from build123d import *

# Parameters (mm, degrees)
F1_DEPTH = 100
F2_DEPTH = 25
F3_DEPTH = 50
F5_DEPTH = 12.5
F6_R     = 15


with BuildPart() as f1:
    # F0 (on Front) → F1 (new body, symmetric)
    with BuildSketch(Plane.XZ):
        Polygon((-50, 25), (-50, -25), (50, -25), (50, 25), (19.234454, 25), (-0.765546, 25), align=None)
    extrude(amount=F1_DEPTH, both=True)

    # F0 (on Front) → F2 (join, symmetric)
    with BuildSketch(Plane.XZ):
        with BuildLine():
            Line((-0.765546, 60), (-0.765546, 25))
            Line((-0.765546, 25), (19.234454, 25))
            Line((19.234454, 25), (19.234454, 60))
            ThreePointArc((19.234454, 60), (37.397461, 98.553935), (78.690689, 109.097654))
            Line((78.690689, 109.097654), (118.690689, 109.097654))
            Line((118.690689, 109.097654), (118.690689, 129.097654))
            Line((118.690689, 129.097654), (80.437767, 129.097654))
            add(Edge.make_bspline(
                [(53.363976, 128.17718), (62.022985, 128.828118), (71.068506, 129.097654), (80.437767, 129.097654)],
                knots=[145.637672, 145.637672, 145.637672, 145.637672, 166.884189, 166.884189, 166.884189, 166.884189], degree=3))
            ThreePointArc((53.363976, 128.17718), (14.412316, 103.526237), (-0.765546, 60))
        make_face()
    extrude(amount=F2_DEPTH, both=True)

    # F0 (on Front) → F3 (join, symmetric)
    with BuildSketch(Plane.XZ):
        Polygon((118.690689, 146.330218), (118.690689, 129.097654), (118.690689, 109.097654), (118.690689, 89.097654), (158.690689, 89.097654), (158.690689, 146.330218), align=None)
    extrude(amount=F3_DEPTH, both=True)

    # F0 (on Front) → F4 (revolve)
    with BuildSketch(Plane.XZ):
        Polygon((118.690689, 146.330218), (118.690689, 129.097654), (118.690689, 109.097654), (118.690689, 89.097654), (158.690689, 89.097654), (158.690689, 146.330218), align=None)
    revolve(axis=Axis((158.690689, 0, 117.713936), (0, 0, 1)))

    # F0 (on Front) → F5 (join, symmetric)
    with BuildSketch(Plane.XZ):
        with BuildLine():
            add(Edge.make_bspline(
                [(-50, 25), (-47.184367, 101.332585), (-5.990596, 123.715224), (53.363976, 128.17718)],
                knots=[0, 0, 0, 0, 145.637672, 145.637672, 145.637672, 145.637672], degree=3))
            Line((-50, 25), (-0.765546, 25))
            Line((-0.765546, 25), (-0.765546, 60))
            ThreePointArc((-0.765546, 60), (14.412316, 103.526237), (53.363976, 128.17718))
        make_face()
    extrude(amount=F5_DEPTH, both=True)

    # F6
    f6_edges = [f1.edges().sort_by_distance(p)[0] for p in [
        (-50, -100, 0),
        (50, -100, 0),
        (50, 100, 0),
        (-50, 100, 0),
    ]]
    fillet(f6_edges, radius=F6_R)


solid = f1.part
The model under review builds one solid part; all positions refer to its coordinate system, in mm. A direction names the side the tool comes from. Round coordinates to 2 decimals unless told otherwise and drop trailing zeros. Order: outer loops, then holes, each group sorted by start corner. A loop starts at its lowest first (then second) coordinate and runs counter-clockwise, first axis right, second up. Notation, with made-up numbers: (-8, 31) -> (-4, 31) arc R32 ccw to (-4, 57) -> close; hole circle Ø3 at (2.5, 51). An arc over 180 degrees is marked (long way). Return JSON: item names as keys, results as strings.
1. Insertion check: P1, Ø6, axis at x = 23.5, z = 60, coming from the -Y side; P2, Ø4, axis at x = 105, y = -20, coming from the -Z side; P3, Ø8, axis at x = 30.5, y = 38, coming from the +Z side; P4, Ø6, axis at x = 9.5, y = 13, coming from the +Z side. Each pin has a flat end and moves straight along its axis. Give the tip position at first contact, or say it passes through.
Answer block:
{"P1": "passes through", "P2": "stops at z = 109.1", "P3": "stops at z = 25", "P4": "stops at z = 120.87"}
2. For L1, parallel to X at y = -38, z = -3.5; L2, parallel to X at y = -21.5, z = 52, list the stretches that pass through material, from the lowest coordinate up. Write a range as [from, to].
Answer block:
{"L1": "x = [-50, 50]", "L2": "x = [-0.77, 19.23]"}
3. Take a section at C-C (x = 165). Write out the cut boundary in (y, z).
Answer block:
{"outline": "(-39.5, 89.1) -> (39.5, 89.1) -> (39.5, 146.33) -> (-39.5, 146.33) -> close"}
4. The part is to be moulded in two halves that separate along X. For faces 6 (the face through (100, 0, 129.098)), 7 (the face through (198.68, -0.88, 117.31)), 8 (the face through (36.925, -0.35, 98.159)), 9 (the face through (98, 0, 109.098)), say which applies: +X half, -X half, draft (parallel to the pull), parting line (faces both ways), or undercut.
Answer block:
{"face 6": "draft", "face 7": "+X half", "face 8": "undercut", "face 9": "undercut"}
5. Take a section at A-A (y = 44). Write out the cut boundary in (x, z).
Answer block:
{"outline": "(-50, -25) -> (50, -25) -> (50, 25) -> (-50, 25) -> close; (118.69, 89.1) -> (158.69, 89.1) -> (158.69, 146.33) -> (118.69, 146.33) -> close"}
6. Take a section at B-B (y = -66). Write out the cut boundary in (x, z).
Answer block:
{"outline": "(-50, -25) -> (50, -25) -> (50, 25) -> (-50, 25) -> close"}
7. For faces 1 (the face through (-1, -1, -25)), 2 (the face through (50, -1, 0)), 3 (the face through (158.691, -45, 117)), 4 (the face through (-17, 12.5, 69)), 5 (the face through (138, 50, 118)), list the 3-axis set-ups (+Z, -Z, +X, -X, +Y, -Y) from which the entire face can be reached by the end or side of a thin tool; tool diameter is ignored.
Answer block:
{"face 1": "-Z, +X, -X, +Y, -Y", "face 2": "-Z, +X, +Y, -Y", "face 3": "+Z, -Z, +X, -Y", "face 4": "+Z, -X, +Y", "face 5": "+Z, -Z, +X, -X, +Y"}
